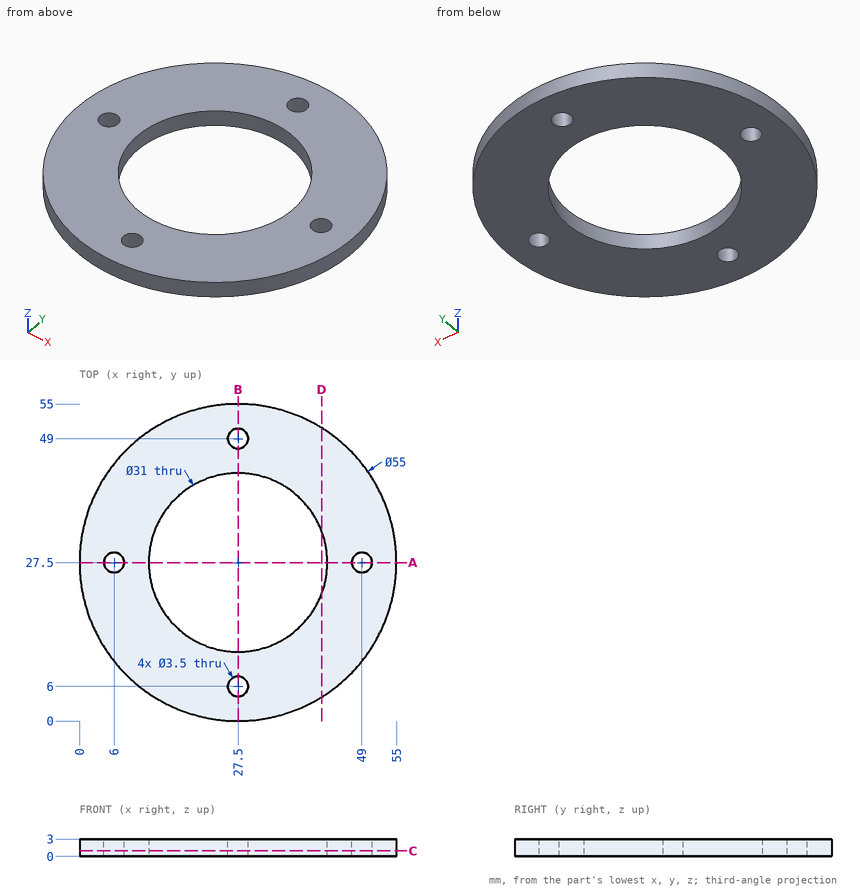
Design review of the part shown in the three views and the two pictorial views. Dimensions are in mm from the part's minimum x, y and z. Coordinates: 2 decimals unless noted, no trailing zeros. Loops run counter-clockwise (first coordinate to the right, second up) from the corner with the lowest first, then second, coordinate; pieces in that order, holes last. Notation, with made-up numbers: (75.5, 5) - (109.5, 5) arc R13 ccw to (109.5, 15) - close; hole circle Ø3 at (1.25, 53.5). An arc over 180 degrees is marked (long way). Use a Markdown table: item, result. Add a question column.
Item 1: We need section D-D (x = 42). Give the boundary of the cut face in (y, z), and give its area (3 significant figures).
Item 2: We need section C-C (z = 0.95). Give the boundary of the cut face in (x, y), and give its area (3 significant figures).
Item 3: We need section A-A (y = 27.5). Give the boundary of the cut face in (x, z).
Item 4: Insertion check: pin 1 Ø3 at (x, y) = (27.5, 49) entering from -Z; pin 2 Ø1 at (x, z) = (17.5, 2.5) entering from +Y. Each pin has a flat end and moves straight along its axis. Give the tip position at first contact, or say it passes through.
Item 5: For line 1 (Y direction, x = 27.5, z = 0.95); line 2 (X direction, y = 27, z = 1.3); line 3 (X direction, y = 49.5, z = 1.8), list the stretches that pass through material, from the lowest coordinate up.
Results list:
| question | item | result |
|---|---|---|
| 1 | outline | (4.13, 0) - (22.02, 0) - (22.02, 3) - (4.13, 3) - close; (32.98, 0) - (50.87, 0) - (50.87, 3) - (32.98, 3) - close |
| 1 | area | 107 mm^2 |
| 2 | outline | circle Ø55 at (27.5, 27.5); hole circle Ø3.5 at (6, 27.5); hole circle Ø31 at (27.5, 27.5); hole circle Ø3.5 at (27.5, 6); hole circle Ø3.5 at (27.5, 49); hole circle Ø3.5 at (49, 27.5) |
| 2 | area | 1,580 mm^2 |
| 3 | outline | (0, 0) - (4.25, 0) - (4.25, 3) - (0, 3) - close; (7.75, 0) - (12, 0) - (12, 3) - (7.75, 3) - close; (43, 0) - (47.25, 0) - (47.25, 3) - (43, 3) - close; (50.75, 0) - (55, 0) - (55, 3) - (50.75, 3) - close |
| 4 | pin 1 | passes through |
| 4 | pin 2 | stops at y = 53.31 |
| 5 | line 1 | y = 0 to 4.25, 7.75 to 12, 43 to 47.25, 50.75 to 55 |
| 5 | line 2 | x = 0 to 4.32, 7.68 to 12.01, 42.99 to 47.32, 50.68 to 55 |
| 5 | line 3 | x = 11 to 25.82, 29.18 to 44 |
